For this review, take the finished solid that the model builds, in its own axes (mm). Face numbers are marked on the shaded views. A direction names the side the tool comes from. Coordinates: 2 decimals unless noted, no trailing zeros. Loops run counter-clockwise (first coordinate to the right, second up) from the corner with the lowest first, then second, coordinate; pieces in that order, holes last. Notation, with made-up numbers: M 81,31 L 116,31 A27 ccw 116,51 Z; hole C 17.25,22 d3. An arc over 180 degrees is marked long. Put each result on its own line as item: value.
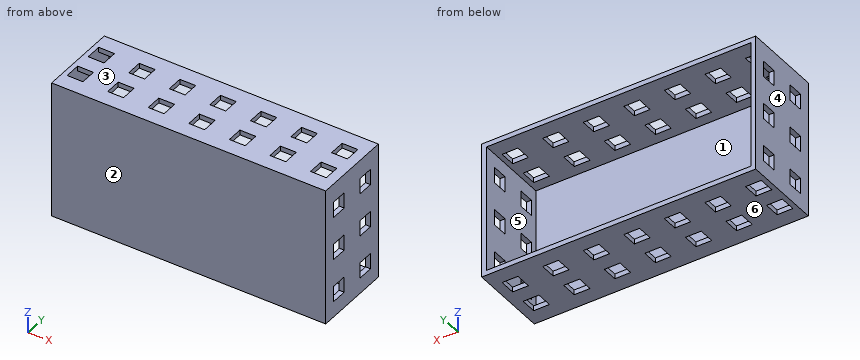
```python
from build123d import *

# Parameters (mm, degrees)
F0_W     = 138.5
F0_H     = 69.5
F1_DEPTH = 40
F2_T     = -2.5
F3_W     = 8
F3_H     = 8
F4_DEPTH = 100
F5_W     = 8
F5_H     = 8
F6_DEPTH = 200


with BuildPart() as f1:
    # F0 (on Front) → F1 (new body)
    with BuildSketch(Plane.XZ):
        with Locations((69.25, 34.75)):
            Rectangle(F0_W, F0_H)
    extrude(amount=F1_DEPTH)

    # F2
    f2_openings = [f1.faces().sort_by_distance(p)[0] for p in [
        (69.25, 0, 34.75),
    ]]
    offset(amount=F2_T, openings=f2_openings)

    # F3 (on face) → F4 (cut)
    with BuildSketch(Plane(origin=(0, 0, 0), x_dir=(1, 0, 0), z_dir=(0, 0, -1))):
        with Locations((6.5, 28)):
            Rectangle(F3_W, F3_H)
        with Locations((27, 28)):
            Rectangle(F3_W, F3_H)
        with Locations((27, 12)):
            Rectangle(F3_W, F3_H)
        with Locations((6.5, 12)):
            Rectangle(F3_W, F3_H)
        with Locations((47.5, 12)):
            Rectangle(F3_W, F3_H)
        with Locations((47.5, 28)):
            Rectangle(F3_W, F3_H)
        with Locations((68, 28)):
            Rectangle(F3_W, F3_H)
        with Locations((68, 12)):
            Rectangle(F3_W, F3_H)
        with Locations((88.5, 12)):
            Rectangle(F3_W, F3_H)
        with Locations((88.5, 28)):
            Rectangle(F3_W, F3_H)
        with Locations((109, 28)):
            Rectangle(F3_W, F3_H)
        with Locations((109, 12)):
            Rectangle(F3_W, F3_H)
        with Locations((129.5, 12)):
            Rectangle(F3_W, F3_H)
        with Locations((129.5, 28)):
            Rectangle(F3_W, F3_H)
    extrude(amount=-F4_DEPTH, mode=Mode.SUBTRACT)

    # F5 (on face) → F6 (cut)
    with BuildSketch(Plane(origin=(0, 0, 0), x_dir=(0, -1, 0), z_dir=(-1, 0, 0))):
        with Locations((10, 12)):
            Rectangle(F5_W, F5_H)
        with Locations((10, 34)):
            Rectangle(F5_W, F5_H)
        with Locations((30, 12)):
            Rectangle(F5_W, F5_H)
        with Locations((30, 34)):
            Rectangle(F5_W, F5_H)
        with Locations((30, 56)):
            Rectangle(F5_W, F5_H)
        with Locations((10, 56)):
            Rectangle(F5_W, F5_H)
    extrude(amount=-F6_DEPTH, mode=Mode.SUBTRACT)


solid = f1.part
```
(1) Wall thickness on line 1 along Z through (x, y) = (96, -30.5); line 2 along X through (y, z) = (-28.5, 16.5); line 3 along Y through (x, z) = (30.5, 42): over which ranges is each line inside the solid? List them lowest first. Write a range as [from, to].
Determined:
line 1: z = [0, 2.5], [67, 69.5]
line 2: x = [0, 2.5], [136, 138.5]
line 3: y = [-40, -37.5]
(2) Add section C-C (y = -10). State how many separate pieces and enclosed holes the cut face has, plus the area to 3 significant figures.
Determined:
separate pieces: 20
enclosed holes: 0
area: 615 mm^2
(3) Add section D-D (z = 25). Write out the cut boundary in (x, y).
Determined:
outline: M 0,-40 L 138.5,-40 L 138.5,0 L 136,0 L 136,-37.5 L 2.5,-37.5 L 2.5,0 L 0,0 Z
(4) Tool access review of the marked faces 1 and 2: name each direction out of +Z, -Z, +X, -X, +Y, -Y from which nothing blocks a thin tool from reaching the whole face with its end or side.
Determined:
face 1: +Y
face 2: +Z, -Z, +X, -X, -Y
(5) Draft analysis for pull direction Z (two halves, no side actions). For the marked faces 3, 4, 5 and 6, state which applies: +Z half, -Z half, draft (parallel to the pull), parting line (faces both ways), or undercut.
Determined:
face 3: +Z half
face 4: draft
face 5: undercut
face 6: -Z half
(6) Add section B-B (z = 14). Write out the cut boundary in (x, y), plus the area to 3 significant figures.
Determined:
outline: M 0,-40 L 138.5,-40 L 138.5,-34 L 136,-34 L 136,-37.5 L 2.5,-37.5 L 2.5,-34 L 0,-34 Z; M 0,-26 L 2.5,-26 L 2.5,-14 L 0,-14 Z; M 0,-6 L 2.5,-6 L 2.5,0 L 0,0 Z; M 136,-26 L 138.5,-26 L 138.5,-14 L 136,-14 Z; M 136,-6 L 138.5,-6 L 138.5,0 L 136,0 Z
area: 454 mm^2
(7) Add section A-A (x = 46). Write out the cut boundary in (y, z), plus the area to 3 significant figures.
Determined:
outline: M -40,0 L -32,0 L -32,2.5 L -37.5,2.5 L -37.5,67 L -32,67 L -32,69.5 L -40,69.5 Z; M -24,0 L -16,0 L -16,2.5 L -24,2.5 Z; M -24,67 L -16,67 L -16,69.5 L -24,69.5 Z; M -8,0 L 0,0 L 0,2.5 L -8,2.5 Z; M -8,67 L 0,67 L 0,69.5 L -8,69.5 Z
area: 281 mm^2
